```python
from build123d import *

# Parameters (mm, degrees)
F0_R     = 2.1
F0_R_2   = 1.6
F1_DEPTH = 1.5
F2_R     = 10


with BuildPart() as f1:
    # F0 (on Top) → F1 (new body)
    with BuildSketch(Plane.XY):
        Polygon((-20.152543, 32.880465), (-32.880465, 20.152543), (-22.5, 5.327702), (-22.5, -5.327702), (-32.880465, -20.152543), (-20.152543, -32.880465), (-5.327702, -22.5), (5.327702, -22.5), (20.152543, -32.880465), (32.880465, -20.152543), (22.5, -5.327702), (22.5, 5.327702), (32.880465, 20.152543), (20.152543, 32.880465), (5.327702, 22.5), (-5.327702, 22.5), align=None)
        with Locations((-21.213203, -21.213203)):
            Circle(F0_R, mode=Mode.SUBTRACT)
        with Locations((-15.25, -15.25)):
            Circle(F0_R_2, mode=Mode.SUBTRACT)
        with Locations((-7.071068, -7.071068)):
            Circle(F0_R, mode=Mode.SUBTRACT)
        with Locations((21.213203, -21.213203)):
            Circle(F0_R, mode=Mode.SUBTRACT)
        with Locations((15.25, -15.25)):
            Circle(F0_R_2, mode=Mode.SUBTRACT)
        with Locations((7.071068, -7.071068)):
            Circle(F0_R, mode=Mode.SUBTRACT)
        with Locations((-7.071068, 7.071068)):
            Circle(F0_R, mode=Mode.SUBTRACT)
        with Locations((-15.25, 15.25)):
            Circle(F0_R_2, mode=Mode.SUBTRACT)
        with Locations((-21.213203, 21.213203)):
            Circle(F0_R, mode=Mode.SUBTRACT)
        with Locations((7.071068, 7.071068)):
            Circle(F0_R, mode=Mode.SUBTRACT)
        with Locations((15.25, 15.25)):
            Circle(F0_R_2, mode=Mode.SUBTRACT)
        with Locations((21.213203, 21.213203)):
            Circle(F0_R, mode=Mode.SUBTRACT)
    extrude(amount=F1_DEPTH)

    # F2
    f2_edges = [f1.edges().sort_by_distance(p)[0] for p in [
        (-32.880465, 20.152543, 0.75),
        (-22.5, 5.327702, 0.75),
        (-22.5, -5.327702, 0.75),
        (-32.880465, -20.152543, 0.75),
        (-20.152543, -32.880465, 0.75),
        (-5.327702, -22.5, 0.75),
        (5.327702, -22.5, 0.75),
        (20.152543, -32.880465, 0.75),
        (32.880465, -20.152543, 0.75),
        (22.5, -5.327702, 0.75),
        (22.5, 5.327702, 0.75),
        (32.880465, 20.152543, 0.75),
        (-20.152543, 32.880465, 0.75),
        (20.152543, 32.880465, 0.75),
        (5.327702, 22.5, 0.75),
        (-5.327702, 22.5, 0.75),
    ]]
    fillet(f2_edges, radius=F2_R)


solid = f1.part
```
Geometry check sheet. Reference: the model listing, model coordinates, mm. A direction names the side the tool comes from. Give positions to 0.01 mm unless a question says otherwise; leave off trailing zeros. Loops run counter-clockwise (first coordinate to the right, second up) from the corner with the lowest first, then second, coordinate; pieces in that order, holes last. Notation, with made-up numbers: M 67,-3.75 L 119,-3.75 A5 cw 119,5.25 Z; hole C 43.5,17 d6. An arc over 180 degrees is marked long. Answer as CSV lines item,"result".
Item 1: Release check for a two-part mould opening along X. For faces 1 (the cylindrical face through (22.95, -5.14, 0.76)), 2 (the cylindrical face through (13.65, -15.18, 0.74)), 3 (the cylindrical face through (6.62, 5.02, 0.74)), 4 (the cylindrical face through (-22.95, -5.14, 0.76)) record: pulls with the +X half, pulls with the -X half, needs draft (parallel to the pull), parting line crosses it, or undercut.
Values:
face 1,"pulls with the +X half"
face 2,"undercut"
face 3,"undercut"
face 4,"pulls with the -X half"
Item 2: Cross-section at D-D on y = -4. Record the cut outline in (x, z).
Values:
outline,"M -22.67,0 L 22.67,0 L 22.67,1.5 L -22.67,1.5 Z"
Item 3: Cross-section at C-C on z = 0.8. Count the separate pieces of the cut face and the enclosed holes in it, and give its area (3 significant figures).
Values:
separate pieces,"1"
enclosed holes,"12"
area,"2,690 mm²"
Item 4: Cross-section at B-B on y = -14.5. Record the cut outline in (x, z).
Values:
outline,"M -28.8,0 L -16.66,0 L -16.66,1.5 L -28.8,1.5 Z; M -13.84,0 L 13.84,0 L 13.84,1.5 L -13.84,1.5 Z; M 16.66,0 L 28.8,0 L 28.8,1.5 L 16.66,1.5 Z"
Item 5: Cross-section at A-A on x = -15. Record the cut outline in (y, z).
Values:
outline,"M -29.03,0 L -16.83,0 L -16.83,1.5 L -29.03,1.5 Z; M -13.67,0 L 13.67,0 L 13.67,1.5 L -13.67,1.5 Z; M 16.83,0 L 29.03,0 L 29.03,1.5 L 16.83,1.5 Z"
Item 6: Material ranges on line 1 (Y direction, x = 15.25, z = 0.95); line 2 (X direction, y = -5.5, z = 0.95); line 3 (X direction, y = -7.5, z = 0.6), recorded low to high.
Values:
line 1,"y = -29.14 to -16.85, -13.65 to 13.65, 16.85 to 29.14"
line 2,"x = -23.07 to -8.46, -5.68 to 5.68, 8.46 to 23.07"
line 3,"x = -24.04 to -9.13, -5.02 to 5.02, 9.13 to 24.04"
Item 7: Access from +Z, -Z, +X, -X, +Y, -Y to the whole of each face (thin tool, end or side, straight path). Record for faces 5 (the flat face through (-26.214, 10.632, 0.74)), 6 (the cylindrical face through (22.976, 5.223, 0.76)), 7 (the flat face through (0, -22.5, 1)).
Values:
face 5,"+Z, -Z, -X"
face 6,"+Z, -Z, +X"
face 7,"+Z, -Z, -Y"
Item 8: Depth check by flat-ended pin: P1, Ø0.8, axis at x = -0.5, z = 1, coming from the -Y side; P2, Ø1.5, axis at x = 15.5, y = 11, coming from the -Z side; P3, Ø4, axis at x = -7.07, y = -7.07, coming from the +Z side; P4, Ø0.8, axis at y = 0.5, z = 1, coming from the +X side. Enter the tip coordinate at first touch or a pass-through.
Values:
P1,"stops at y = -22.5"
P2,"stops at z = 0"
P3,"passes through"
P4,"stops at x = 22.5"
